from build123d import *

# Parameters (mm, degrees)
BOSS_EXTRUDE1_DEPTH         = 1.5
BOSS_EXTRUDE1_DEPTH_BACK    = 1.5
HOLDER_RING_R               = 4.875
HOLDER_RING_R_2             = 2.375
M2X0_25_TAPPED_HOLE1_REACH  = 13.016
M2X0_25_TAPPED_HOLE1_BORE_R = 0.875
MIRROR1_START               = -2.389401654
MIRROR1_DEPTH               = 7.264401636


# Read off the part's stored shape, not the designer's step: Mirror1
with BuildPart() as part:
    # holder_ring → Boss-Extrude1 (new, two sides: drawn at the far end of the back side and taken through both)
    with BuildSketch(Plane(origin=(0, 0, 0), x_dir=(1, 0, 0), z_dir=(0, 1, 0)).offset(-BOSS_EXTRUDE1_DEPTH_BACK)):
        with Locations(Location((0, 0, 0), (0, 0, 270))):
            Circle(HOLDER_RING_R)
        with Locations(Location((0, 0, 0), (0, 0, 270))):
            Circle(HOLDER_RING_R_2, mode=Mode.SUBTRACT)
    extrude(amount=BOSS_EXTRUDE1_DEPTH + BOSS_EXTRUDE1_DEPTH_BACK)

    # M2x0.25 Tapped Hole1 bore (on position points) → M2x0.25 Tapped Hole1 (cut, up to next)
    with BuildSketch(Plane(origin=(0.02757507, 0.000556894, -4.874922011), x_dir=(-0.999984002302, 0, -0.005656424646), z_dir=(0.005656424646, 0, -0.999984002302)), mode=Mode.PRIVATE) as m2x0_25_tapped_hole1_sk1:
        Circle(M2X0_25_TAPPED_HOLE1_BORE_R)
    m2x0_25_tapped_hole1_tool1 = extrude(m2x0_25_tapped_hole1_sk1.sketch, amount=-M2X0_25_TAPPED_HOLE1_REACH, mode=Mode.PRIVATE) & part.part
    add(m2x0_25_tapped_hole1_tool1.solids().sort_by_distance((0.027575, 0.000557, -4.874922))[0], mode=Mode.SUBTRACT)

    # Mirror1 outline → Mirror1 (cut)
    with BuildSketch(Plane(origin=(0, 0, 0), x_dir=(0.99998400230215, 0, -0.00565642464579779), z_dir=(0.00565642464579779, 0, 0.99998400230215)).offset(MIRROR1_START)):
        with BuildLine():
            ThreePointArc((0.013515687, -0.874338715), (0.875, 0.000556894), (0.013515687, 0.875452503))
            ThreePointArc((0.013515687, 0.875452503), (-0.875, 0.000556894), (0.013515687, -0.874338715))
        make_face()
    extrude(amount=MIRROR1_DEPTH, mode=Mode.SUBTRACT)


solid = part.part
Part model, mm, in its own coordinate system. Coordinates: 2 decimals unless noted, no trailing zeros. Write each loop counter-clockwise with the first axis right and the second up, starting at its lowest first coordinate (ties: lowest second). Pieces come first, ordered by that corner, then holes. Notation, with made-up numbers: M 62,77 L 85,77 A9 cw 85,88 Z; hole C -24,22.5 d7. An arc over 180 degrees is marked long. Return JSON: item names as keys, results as strings.
1. Flat gauge pins, fed straight in: pin 1 Ø1 at (x, y) = (-3.5, -0.5) entering from +Z; pin 2 Ø1 at (x, y) = (-3, -0.5) entering from +Z. Where does each tip first touch, or does it go through?
Determined:
{"pin 1": "z = 3.84", "pin 2": "z = 4.19"}
2. Saw through at C-C, the plane y = 1.3. Write the cut outline in (x, z) (3 decimals), then the cut area to 3 significant figures.
Determined:
{"outline": "C 0,0 d9.75; hole C 0,0 d4.75", "area": "56.9 mm²"}
3. Saw through at D-D, the plane x = -3. Write the cut outline in (y, z).
Determined:
{"outline": "M -1.5,-3.84 L 1.5,-3.84 L 1.5,3.84 L -1.5,3.84 Z"}
4. Saw through at B-B, the plane y = -0.4. Write the cut outline in (x, z) (3 decimals), then the cut area to 3 significant figures.
Determined:
{"outline": "M -0.791,-2.385 L -0.791,-2.24 A2.375 cw -0.765,2.248 L -0.751,4.817 A4.875 ccw -0.751,-4.817 L -0.764,-2.385 Z; M 0.791,-2.24 L 0.805,-4.808 A4.875 ccw 0.805,4.808 L 0.791,2.24 A2.375 cw Z", "area": "49.1 mm²"}
5. Saw through at A-A, the plane z = 0. Write the cut outline in (x, y) (3 decimals), then the cut area to 3 significant figures.
Determined:
{"outline": "M -4.875,-1.5 L -2.375,-1.5 L -2.375,1.5 L -4.875,1.5 Z; M 2.375,-1.5 L 4.875,-1.5 L 4.875,1.5 L 2.375,1.5 Z", "area": "15.0 mm²"}
6. Probe L1, parallel to X at y = -0.35, z = 0 (3 decimals); L2, parallel to Z at x = -1, y = 0.35; L3, parallel to X at y = 1.15, z = 0.75. List the from-to ranges inside material, lowest first.
Determined:
{"L1": "-4.875 to -2.375, 2.375 to 4.875", "L2": "-4.77 to -2.15, 2.15 to 4.77", "L3": "-4.82 to -2.25, 2.25 to 4.82"}
7. Pull direction X, two halves, no side cores. Call faces 1 (the face through (0.894, 0.039, -3.555)), 2 (the face through (1.46, -0.02, 4.65)): pulls with the +X half, pulls with the -X half, needs draft (parallel to the pull), parting line crosses it, or undercut.
Determined:
{"face 1": "undercut", "face 2": "parting line crosses it"}
